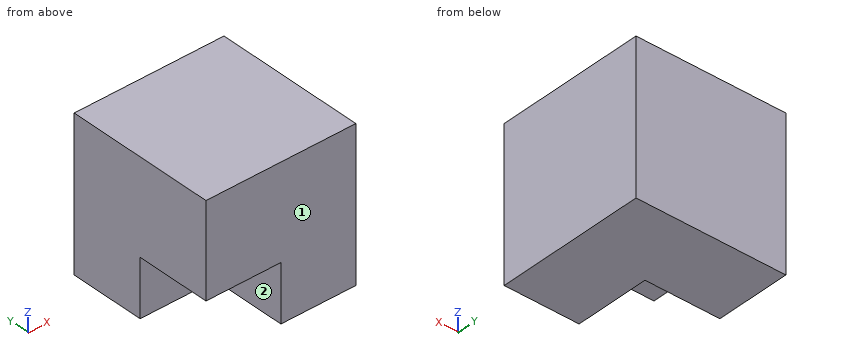
```python
from build123d import *

# Parameters (mm, degrees)
F0_W     = 50.8
F0_H     = 50.8
F1_DEPTH = 50.8
F2_W     = 25.4
F2_H     = 25.4
F3_DEPTH = 25.4
F4_W     = 25.4
F4_H     = 25.4
F5_DEPTH = 25.4
F6_W     = 25.4
F6_H     = 19.28642
F7_DEPTH = 25.4


with BuildPart() as f1:
    # F0 (on Front) → F1 (new body)
    with BuildSketch(Plane.XZ):
        with Locations((-25.4, 25.4)):
            Rectangle(F0_W, F0_H)
    extrude(amount=F1_DEPTH)

    # F2 (on Front) → F3 (cut)
    with BuildSketch(Plane.XZ):
        with Locations((-37.521074, 12.7)):
            Rectangle(F2_W, F2_H)
    extrude(amount=-F3_DEPTH, mode=Mode.SUBTRACT)

    # F4 (on Front) → F5 (cut)
    with BuildSketch(Plane.XZ):
        with Locations((-37.33012, 12.7)):
            Rectangle(F4_W, F4_H)
    extrude(amount=-F5_DEPTH, mode=Mode.SUBTRACT)

    # F6 (on face) → F7 (cut)
    with BuildSketch(Plane.XZ.offset(50.8)):
        with Locations((-38.1, 9.64321)):
            Rectangle(F6_W, F6_H)
    extrude(amount=-F7_DEPTH, mode=Mode.SUBTRACT)


solid = f1.part
```
Verification items for the finished model (mm, model axes). Face numbers are marked on the shaded views. A direction names the side the tool comes from. Round coordinates to 2 decimals unless told otherwise and drop trailing zeros. Write each loop counter-clockwise with the first axis right and the second up, starting at its lowest first coordinate (ties: lowest second). Pieces come first, ordered by that corner, then holes. Notation, with made-up numbers: (20.5, -40) -> (27.5, -40) arc R22 ccw to (27.5, -34) -> close; hole circle Ø11 at (67, 79.5). An arc over 180 degrees is marked (long way). Write each question's results on one line, items separated by ' | '. Start each with the question number.
1. Depth check by flat-ended pin: P1, Ø1.5, axis at y = -28.5, z = 15.5, coming from the -X side; P2, Ø4, axis at x = -39.5, y = -39, coming from the -Z side. Enter the tip coordinate at first touch or a pass-through.
2. Material ranges on probe 1 along X at (y, z) = (-27, 4.5); probe 2 along Z at (x, y) = (-29, -48), recorded low to high. Write a range as from..to.
3. Cross-section at A-A (y = -34). Enter the section's corners in (x, z), then the cut area to 3 significant figures.
4. Cross-section at B-B (z = 10). Enter the section's corners in (x, y), then the cut area to 3 significant figures.
5. Set-up check for the marked faces 1 and 2: record each of +Z, -Z, +X, -X, +Y, -Y from which the full face is reachable in a straight line by a thin tool's end or side.
Solutions:
1) P1: stops at x = -25.4 | P2: stops at z = 19.29
2) probe 1: x = -25.4..0 | probe 2: z = 19.29..50.8
3) outline: (-50.8, 19.29) -> (-25.4, 19.29) -> (-25.4, 0) -> (0, 0) -> (0, 50.8) -> (-50.8, 50.8) -> close | area: 2,090 mm2
4) outline: (-50.8, -25.4) -> (-25.4, -25.4) -> (-25.4, -50.8) -> (0, -50.8) -> (0, 0) -> (-50.8, 0) -> close | area: 1,940 mm2
5) face 1: +Z, -Z, +X, -X, -Y | face 2: -Z, -X, -Y
